from build123d import *

# Parameters (mm, degrees)
SKETCH_R        = 24
SKETCH_R_2      = 15
PAD_DEPTH       = 18
SKETCH001_R     = 75
PAD001_DEPTH    = 30
PAD001_TAPER    = 25
SKETCH002_R     = 40
POCKET_DEPTH    = 20
POCKET_FACE23_R = 24
POCKET001_DEPTH = 30.001


with BuildPart() as part:
    # Sketch → Pad (new body)
    with BuildSketch(Plane.XY):
        with BuildLine():
            ThreePointArc((-72.230677, 20.192308), (-51.220332, -54.785742), (25, -70.710678))
            Line((25, -115), (25, -70.710678))
            ThreePointArc((10, -130), (20.606602, -125.606602), (25, -115))
            Line((-45, -130), (10, -130))
            ThreePointArc((-45, -130), (-75, -160), (-45, -190))
            Line((60, -190), (-45, -190))
            ThreePointArc((60, -190), (70.606602, -185.606602), (75, -175))
            Line((75, 0), (75, -175))
            ThreePointArc((75, 0), (74.304444, 10.190663), (72.230677, 20.192308))
            Line((38.523028, 140.769231), (72.230677, 20.192308))
            ThreePointArc((38.523028, 140.769231), (0, 170), (-38.523028, 140.769231))
            Line((-38.523028, 140.769231), (-72.230677, 20.192308))
        make_face()
        Circle(SKETCH_R, mode=Mode.SUBTRACT)
        with Locations((0, 130)):
            Circle(SKETCH_R_2, mode=Mode.SUBTRACT)
        with BuildLine():
            ThreePointArc((-45, -147), (-58, -160), (-45, -173))
            Line((-45, -173), (19, -173))
            ThreePointArc((19, -173), (32, -160), (19, -147))
            Line((-45, -147), (19, -147))
        make_face(mode=Mode.SUBTRACT)
    extrude(amount=PAD_DEPTH)

    # Sketch001 (on Face20 of Pad) → Pad001 (join)
    with BuildSketch(Plane.XY.offset(18)):
        Circle(SKETCH001_R)
    extrude(amount=PAD001_DEPTH, taper=PAD001_TAPER)

    # Sketch002 (on Face24 of Pad001) → Pocket (cut)
    with BuildSketch(Plane.XY.offset(48)):
        Circle(SKETCH002_R)
    extrude(amount=-POCKET_DEPTH, mode=Mode.SUBTRACT)

    # Pocket Face23 → Pocket001 (cut, through all)
    with BuildSketch(Plane(origin=(0, 0, 18), x_dir=(0, -1, 0), z_dir=(0, 0, -1))):
        Circle(POCKET_FACE23_R)
    extrude(amount=-POCKET001_DEPTH, mode=Mode.SUBTRACT)


solid = part.part
Work out the finished part from the listing and answer in its coordinate system (mm). A direction names the side the tool comes from. Coordinates: 2 decimals unless noted, no trailing zeros. Write each loop counter-clockwise with the first axis right and the second up, starting at its lowest first coordinate (ties: lowest second). Pieces come first, ordered by that corner, then holes. Notation, with made-up numbers: M 42.5,53.5 L 46.5,53.5 A12 ccw 46.5,65.5 Z; hole C 14.25,-2 d4. An arc over 180 degrees is marked long. Use one line per item in the form item = value. Start each with the question number.
1. The part is cut by section B-B (z = 10). Give the vertices of the cut face in (x, y), plus the area to 3 significant figures.
2. The part is cut by section A-A (y = -160). Give the vertices of the cut face in (x, z).
3. Straight lines are drawn through the part: probe 1 along Y at (x, z) = (0, 12.5); probe 2 along X at (y, z) = (0, 10.25); probe 3 along Z at (x, y) = (-50, 64). For each, find the intervals that lie inside material, in ascending order. Write a range as from..to.
4. The mould has two halves that part along Y. Classify faces 4 (the face through (8, -190, 9)), 5 (the face through (0.727, 169.993, 8.874)), 6 (the face through (-58, -160, 9)): released by +Y, released by -Y, zero draft, split by the parting line, or undercut.
5. The part is cut by section C-C (x = 0). Give the vertices of the cut face in (y, z), plus the area to 3 significant figures.
6. Each of these flat-tipped pins is pushed along its axis until it touches: P1, Ø14.5, axis at x = 0, z = 8.5, coming from the +Y side; P2, Ø1, axis at y = -127.5, z = 9, coming from the -X side; P3, Ø10, axis at x = -50.5, z = 42.5, coming from the +Y side. Where does it stop, or does it pass through?
7. The part is cut by section D-D (z = 24). Give the vertices of the cut face in (x, y).
8. A tool of negligible diameter and unlimited length cuts with its end or side. For faces 1 (the face through (20.49, -125.72, 8.87)), 2 (the face through (-13, -173, 9)), 3 (the face through (16, -136, 18)), from which of +Z, -Z, +X, -X, +Y, -Y can it reach the whole face along a straight path? Write none if from no direction.
Evaluation:
q1.outline = M -72.23,20.19 A75 ccw 25,-70.71 L 25,-115 A15 cw 10,-130 L -45,-130 A30 ccw -45,-190 L 60,-190 A15 ccw 75,-175 L 75,0 A75 ccw 72.23,20.19 L 38.52,140.77 A40 ccw -38.52,140.77 Z; hole M -45,-173 L 19,-173 A13 ccw 19,-147 L -45,-147 A13 ccw Z; hole C 0,0 d48; hole C 0,130 d30
q1.area = 34,700 mm^2
q2.outline = M -75,0 L -58,0 L -58,18 L -75,18 Z; M 32,0 L 75,0 L 75,18 L 32,18 Z
q3.probe_1 = -190..-173, -147..-130, -75..-24, 24..115, 145..170
q3.probe_2 = -75..-24, 24..75
q3.probe_3 = 0..18
q4.face_4 = released by -Y
q4.face_5 = released by +Y
q4.face_6 = undercut
q5.outline = M -190,0 L -173,0 L -173,18 L -190,18 Z; M -147,0 L -130,0 L -130,18 L -147,18 Z; M -75,0 L -24,0 L -24,28 L -40,28 L -40,48 L -61.01,48 L -75,18 Z; M 24,0 L 115,0 L 115,18 L 75,18 L 61.01,48 L 40,48 L 40,28 L 24,28 Z; M 145,0 L 170,0 L 170,18 L 145,18 Z
q5.area = 5,620 mm^2
q6.P1 = 170
q6.P2 = 17.48
q6.P3 = 45.39
q7.outline = C 0,0 d144.4; hole C 0,0 d48
q8.face_1 = +Z, -Z, -X
q8.face_2 = +Z, -Z
q8.face_3 = +Z, +X, -Y
